Print and shaded views of the part. All mm, measured from the part's lowest x, y and z. A direction names the side the tool comes from. Round coordinates to 2 decimals unless told otherwise and drop trailing zeros. Loops run counter-clockwise (first coordinate to the right, second up) from the corner with the lowest first, then second, coordinate; pieces in that order, holes last. Notation, with made-up numbers: (8, 11.5) -> (52, 11.5) arc R22 cw to (52, 49.5) -> close; hole circle Ø9 at (44.25, 48.25). An arc over 180 degrees is marked (long way). Use a Markdown table: item, result.
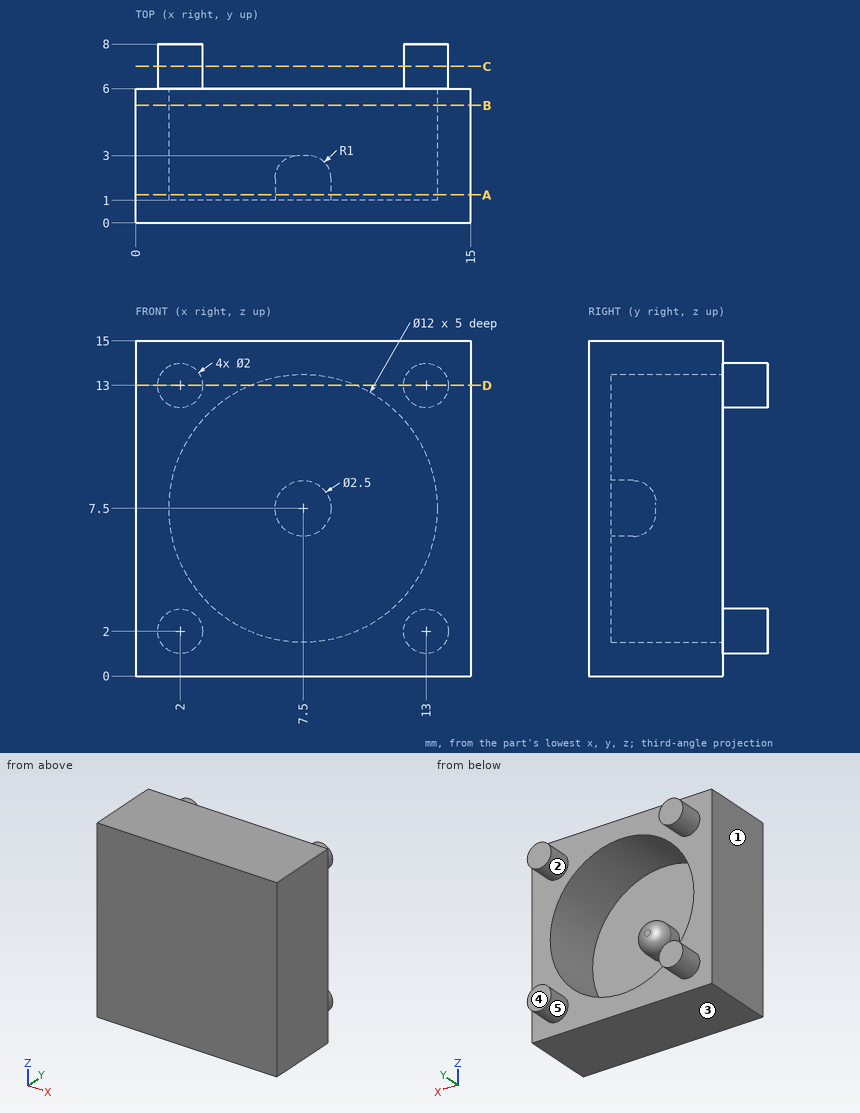
Q1. Pull direction X, two halves, no side cores. Call the marked faces 1, 2 and 3: released by +X, released by -X, zero draft, split by the parting line, or undercut.
Results list:
| item | result |
|---|---|
| face 1 | released by -X |
| face 2 | undercut |
| face 3 | zero draft |
Q2. Band-saw the part on A-A, the plane y = 1.25. Give the cut face in (x, z), plus the area to 3 significant figures.
Results list:
| item | result |
|---|---|
| outline | (0, 0) -> (15, 0) -> (15, 15) -> (0, 15) -> close; circle Ø2.5 at (7.5, 7.5); hole circle Ø12 at (7.5, 7.5) |
| area | 117 mm² |
Q3. Band-saw the part on D-D, the plane z = 13. Give the cut face in (x, y), plus the area to 3 significant figures.
Results list:
| item | result |
|---|---|
| outline | (0, 0) -> (15, 0) -> (15, 6) -> (14, 6) -> (14, 8) -> (12, 8) -> (12, 6) -> (9.9, 6) -> (9.9, 1) -> (5.1, 1) -> (5.1, 6) -> (3, 6) -> (3, 8) -> (1, 8) -> (1, 6) -> (0, 6) -> close |
| area | 74.0 mm² |
Q4. Drill centre lines: L1, parallel to Z at x = 7.75, y = 3.5; L2, parallel to X at y = 4.7, z = 7.5; L3, parallel to Y at x = 1, z = 1.5. Where is each one in solid material? Low to high. Write a range as from..to.
Results list:
| item | result |
|---|---|
| L1 | z = 0..1.51, 13.49..15 |
| L2 | x = 0..1.5, 13.5..15 |
| L3 | y = 0..6 |
Q5. Band-saw the part on B-B, the plane y = 5.25. Give the cut face in (x, z).
Results list:
| item | result |
|---|---|
| outline | (0, 0) -> (15, 0) -> (15, 15) -> (0, 15) -> close; hole circle Ø12 at (7.5, 7.5) |
Q6. Band-saw the part on C-C, the plane y = 7. Give the cut face in (x, z), plus the area to 3 significant figures.
Results list:
| item | result |
|---|---|
| outline | circle Ø2 at (2, 2); circle Ø2 at (2, 13); circle Ø2 at (13, 2); circle Ø2 at (13, 13) |
| area | 12.6 mm² |
Q7. Tool access for the marked faces 4 and 5: list every direction of +Z, -Z, +X, -X, +Y, -Y with a clear straight run to the whole face (end or side of a thin tool).
Results list:
| item | result |
|---|---|
| face 4 | +Z, -Z, +X, -X, +Y |
| face 5 | +Y |
